from build123d import *

# Parameters (mm, degrees)
F0_R     = 1.5
F0_W     = 5
F0_H     = 3
F0_W_2   = 41
F0_H_2   = 20
F1_DEPTH = 3


with BuildPart() as f1:
    # F0 (on Top) → F1 (new body)
    with BuildSketch(Plane.XY):
        with BuildLine():
            Line((245, 160), (5, 160))
            ThreePointArc((5, 160), (1.4644660941, 158.5355339059), (0, 155))
            Line((0, 155), (0, 5))
            ThreePointArc((0, 5), (1.4644660941, 1.4644660941), (5, 0))
            Line((5, 0), (245, 0))
            ThreePointArc((245, 0), (248.5355339059, 1.4644660941), (250, 5))
            Line((250, 5), (250, 155))
            ThreePointArc((250, 155), (248.5355339059, 158.5355339059), (245, 160))
        make_face()
        with Locations((20, 5)):
            Circle(F0_R, mode=Mode.SUBTRACT)
        with Locations((212.5, 10)):
            Rectangle(F0_W, F0_H, mode=Mode.SUBTRACT)
        with Locations((220, 10)):
            Circle(F0_R, mode=Mode.SUBTRACT)
        with Locations((227.5, 10)):
            Rectangle(F0_W, F0_H, mode=Mode.SUBTRACT)
        with Locations((195, 39)):
            Circle(F0_R, mode=Mode.SUBTRACT)
        with Locations((225, 39)):
            Circle(F0_R, mode=Mode.SUBTRACT)
        with Locations((9.9999278665, 70)):
            Circle(F0_R, mode=Mode.SUBTRACT)
        with Locations((24.9999278665, 70)):
            Circle(F0_R, mode=Mode.SUBTRACT)
        with Locations((9.9999278665, 80)):
            Circle(F0_R, mode=Mode.SUBTRACT)
        with Locations((24.9999278665, 80)):
            Circle(F0_R, mode=Mode.SUBTRACT)
        with Locations((9.9999278665, 90)):
            Circle(F0_R, mode=Mode.SUBTRACT)
        with Locations((24.9999278665, 90)):
            Circle(F0_R, mode=Mode.SUBTRACT)
        with Locations((46.5, 75)):
            Circle(F0_R, mode=Mode.SUBTRACT)
        with Locations((46.5, 85)):
            Circle(F0_R, mode=Mode.SUBTRACT)
        with Locations((70, 80)):
            Rectangle(F0_W_2, F0_H_2, mode=Mode.SUBTRACT)
        with Locations((93.5, 75)):
            Circle(F0_R, mode=Mode.SUBTRACT)
        with Locations((93.5, 85)):
            Circle(F0_R, mode=Mode.SUBTRACT)
        with Locations((20, 155)):
            Circle(F0_R, mode=Mode.SUBTRACT)
        with Locations((195, 59)):
            Circle(F0_R, mode=Mode.SUBTRACT)
        with Locations((225, 59)):
            Circle(F0_R, mode=Mode.SUBTRACT)
        with Locations((195, 101)):
            Circle(F0_R, mode=Mode.SUBTRACT)
        with Locations((195, 121)):
            Circle(F0_R, mode=Mode.SUBTRACT)
        with Locations((225, 101)):
            Circle(F0_R, mode=Mode.SUBTRACT)
        with Locations((225, 121)):
            Circle(F0_R, mode=Mode.SUBTRACT)
        with Locations((212.5, 150)):
            Rectangle(F0_W, F0_H, mode=Mode.SUBTRACT)
        with Locations((220, 150)):
            Circle(F0_R, mode=Mode.SUBTRACT)
        with Locations((227.5, 150)):
            Rectangle(F0_W, F0_H, mode=Mode.SUBTRACT)
    extrude(amount=F1_DEPTH)


solid = f1.part
Part model, mm, in its own coordinate system. Give positions to 0.01 mm unless a question says otherwise; leave off trailing zeros. Loops run counter-clockwise (first coordinate to the right, second up) from the corner with the lowest first, then second, coordinate; pieces in that order, holes last. Notation, with made-up numbers: (50.25, -23.5) -> (93.25, -23.5) arc R34 cw to (93.25, 12.5) -> close; hole circle Ø11 at (-33, 8.25). An arc over 180 degrees is marked (long way). Write each question's results on one line, items separated by ' | '. Start each with the question number.
Q1. Band-saw the part on A-A on x = 69.5. List the corners of the cut face in (y, z).
Q2. Wall check: L1, parallel to X at y = 121, z = 1.2; L2, parallel to Y at x = 20, z = 1.85; L3, parallel to X at y = 75, z = 1.1. Give the ranges that are in metal, low to high.
Q3. Band-saw the part on B-B on z = 1.1. Count the separate pieces of the cut face and the enclosed holes in it, plus the area to 3 significant figures.
Results are:
1) outline: (0, 0) -> (70, 0) -> (70, 3) -> (0, 3) -> close; (90, 0) -> (160, 0) -> (160, 3) -> (90, 3) -> close
2) L1: x = 0 to 193.5, 196.5 to 223.5, 226.5 to 250 | L2: y = 0 to 3.5, 6.5 to 153.5, 156.5 to 160 | L3: x = 0 to 45, 48 to 49.5, 90.5 to 92, 95 to 250
3) separate pieces: 1 | enclosed holes: 27 | area: 38,900 mm²
